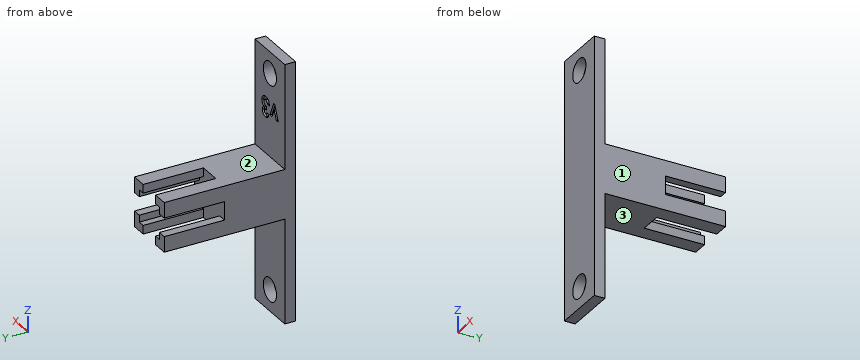
```python
from build123d import *

# Parameters (mm, degrees)
BOSS_EXTRUDE1_DEPTH   = 17.78
BOSS_EXTRUDE1_2_DEPTH = 17.78
BOSS_EXTRUDE1_3_DEPTH = 17.78
BOSS_EXTRUDE1_4_DEPTH = 17.78
SKETCH2_W             = 15.58
SKETCH2_H             = 14.58
BOSS_EXTRUDE2_DEPTH   = 17.78
SKETCH3_W             = 15.58
SKETCH3_H             = 76.2
SKETCH3_R             = 3.429
BOSS_EXTRUDE3_DEPTH   = 3.175
CUT_EXTRUDE3_DEPTH    = 0.635


with BuildPart() as part:
    # Sketch1 → Boss-Extrude1 (new body)
    with BuildSketch(Plane(origin=(0, 0, 0), x_dir=(1, 0, 0), z_dir=(0, 1, 0))):
        Polygon((-5.25, 4.75), (-5.25, 2.718), (-7.79, 2.718), (-7.79, 7.29), (-3.218, 7.29), (-3.218, 4.75), align=None)
    extrude(amount=BOSS_EXTRUDE1_DEPTH)



with BuildPart() as body_2:
    # Sketch1 → Boss-Extrude1 2 (new body)
    with BuildSketch(Plane(origin=(0, 0, 0), x_dir=(1, 0, 0), z_dir=(0, 1, 0))):
        Polygon((7.79, 2.718), (7.79, 7.29), (3.218, 7.29), (3.218, 4.75), (5.25, 4.75), (5.25, 2.718), align=None)
    extrude(amount=BOSS_EXTRUDE1_2_DEPTH)


with BuildPart() as body_3:
    # Sketch1 → Boss-Extrude1 3 (new body)
    with BuildSketch(Plane(origin=(0, 0, 0), x_dir=(1, 0, 0), z_dir=(0, 1, 0))):
        Polygon((5.25, -2.718), (7.79, -2.718), (7.79, -7.29), (3.218, -7.29), (3.218, -4.75), (5.25, -4.75), align=None)
    extrude(amount=BOSS_EXTRUDE1_3_DEPTH)


with BuildPart() as body_4:
    # Sketch1 → Boss-Extrude1 4 (new body)
    with BuildSketch(Plane(origin=(0, 0, 0), x_dir=(1, 0, 0), z_dir=(0, 1, 0))):
        Polygon((-5.25, -2.718), (-7.79, -2.718), (-7.79, -7.29), (-3.218, -7.29), (-3.218, -4.75), (-5.25, -4.75), align=None)
    extrude(amount=BOSS_EXTRUDE1_4_DEPTH)


with BuildPart() as part_1:
    add(part.part)

    add(body_2.part)  # Boss-Extrude2 merges body 2

    add(body_3.part)  # Boss-Extrude2 merges body 3

    add(body_4.part)  # Boss-Extrude2 merges body 4
    # Sketch2 → Boss-Extrude2 (add)
    with BuildSketch(Plane(origin=(0, 0, 0), x_dir=(-1, 0, 0), z_dir=(0, -1, 0))):
        Rectangle(SKETCH2_W, SKETCH2_H)
    extrude(amount=BOSS_EXTRUDE2_DEPTH)

    # Sketch3 → Boss-Extrude3 (add)
    with BuildSketch(Plane(origin=(0, -17.78, 0), x_dir=(-1, 0, 0), z_dir=(0, -1, 0))):
        Rectangle(SKETCH3_W, SKETCH3_H)
        with Locations(Location((0, 31.75, 0), (0, 0, 90))):
            Circle(SKETCH3_R, mode=Mode.SUBTRACT)
        with Locations(Location((0, -31.75, 0), (0, 0, 270))):
            Circle(SKETCH3_R, mode=Mode.SUBTRACT)
    extrude(amount=BOSS_EXTRUDE3_DEPTH)

    # Sketch5 → Cut-Extrude3 (cut)
    with BuildSketch(Plane(origin=(0, -17.78, 0), x_dir=(1, 0, 0), z_dir=(0, 1, 0))):
        Polygon((-4.402938034, -19.56265828), (-3.33951656, -19.56265828), (-2.238782051, -22.073125862), (-1.138047543, -19.56265828), (-0.074626068, -19.56265828), (-1.937945713, -23.816344178), (-2.539618389, -23.816344178), align=None)
        with BuildLine():
            Line((1.60446047, -19.413406143), (0.559695513, -19.413406143))
            add(Edge.make_bspline(
                [(0.559695513, -19.413406143), (0.567071951, -19.36118207), (0.581532969, -19.258800234), (0.616136251, -19.110576841), (0.65752551, -18.969976808), (0.709197886, -18.837445387), (0.769801176, -18.712746497), (0.838719113, -18.59545223), (0.916696725, -18.486066037), (0.976467391, -18.42017136), (1.006285891, -18.387297703)],
                knots=[0, 0, 0, 0, 1.111473889, 2.178970933, 3.205615836, 4.199322666, 5.174200091, 6.12565194, 7.064921805, 8, 8, 8, 8], degree=3))
            add(Edge.make_bspline(
                [(1.006285891, -18.387297703), (1.049295125, -18.343923295), (1.134061806, -18.258436894), (1.275716871, -18.148938257), (1.424197539, -18.054174633), (1.582481657, -17.979045347), (1.748106202, -17.918236894), (1.922388279, -17.877391718), (2.104615709, -17.850290583), (2.228963005, -17.847621027), (2.292419538, -17.846258707)],
                knots=[0, 0, 0, 0, 1.01925491, 2.00884431, 2.983262333, 3.955970413, 4.92937149, 5.924503185, 6.940838805, 8, 8, 8, 8], degree=3))
            add(Edge.make_bspline(
                [(2.292419538, -17.846258707), (2.34883566, -17.847590582), (2.459738389, -17.850208778), (2.622737494, -17.871226235), (2.778143501, -17.908088515), (2.927599095, -17.956285119), (3.068906271, -18.021864654), (3.205183817, -18.097988535), (3.332624133, -18.19135764), (3.451525404, -18.296855331), (3.5607589, -18.410961412), (3.655355585, -18.532931428), (3.736682053, -18.65950728), (3.803684306, -18.791740573), (3.855199933, -18.929855061), (3.890953306, -19.073052878), (3.914354757, -19.221018044), (3.916686153, -19.321587975), (3.91786859, -19.372595012)],
                knots=[0, 0, 0, 0, 1.091422571, 2.145516843, 3.172569842, 4.178562979, 5.178154469, 6.181868002, 7.194278174, 8.227918432, 9.254613415, 10.245994977, 11.209837596, 12.161663635, 13.10878368, 14.055455738, 15.013766427, 16, 16, 16, 16], degree=3))
            add(Edge.make_bspline(
                [(3.91786859, -19.372595012), (3.915442158, -19.435762981), (3.910665261, -19.56012129), (3.871467362, -19.742128915), (3.810111989, -19.916160685), (3.721478187, -20.079781634), (3.610663359, -20.232546477), (3.474697276, -20.369347828), (3.317452606, -20.492330546), (3.199406937, -20.558421473), (3.138959001, -20.592264817)],
                knots=[0, 0, 0, 0, 0.992805628, 1.954529043, 2.915727527, 3.886831945, 4.871318353, 5.87440735, 6.911542536, 8, 8, 8, 8], degree=3))
            add(Edge.make_bspline(
                [(3.138959001, -20.592264817), (3.180449537, -20.605887034), (3.26197658, -20.632654079), (3.377857468, -20.68537147), (3.488046952, -20.742982841), (3.590647607, -20.809912067), (3.686679921, -20.883452827), (3.775558471, -20.964233774), (3.857814283, -21.052078768), (3.932104567, -21.147470922), (3.998040097, -21.248884626), (4.057200536, -21.353977283), (4.105892876, -21.464342641), (4.14714135, -21.578720254), (4.178545589, -21.698138088), (4.20065698, -21.822133409), (4.213437907, -21.950423374), (4.215387216, -22.037339748), (4.216372863, -22.081288088)],
                knots=[0, 0, 0, 0, 1.059543567, 2.081955587, 3.086750234, 4.076226789, 5.052108497, 6.020845489, 6.989030705, 7.970690546, 8.952259656, 9.923888338, 10.895517021, 11.877585046, 12.873342345, 13.889638361, 14.932918083, 16, 16, 16, 16], degree=3))
            add(Edge.make_bspline(
                [(4.216372863, -22.081288088), (4.214374823, -22.145874304), (4.210435096, -22.273225169), (4.18538815, -22.460799959), (4.13875525, -22.639635857), (4.077407087, -22.811790639), (3.995575297, -22.975041849), (3.899273036, -23.13313588), (3.780898209, -23.280590074), (3.649344914, -23.421302739), (3.503247311, -23.549232393), (3.344853741, -23.660141646), (3.177647143, -23.755321519), (3.00056965, -23.832591251), (2.81368278, -23.892097783), (2.61740309, -23.935111847), (2.410905865, -23.961428562), (2.269955352, -23.964187371), (2.19797092, -23.965596314)],
                knots=[0, 0, 0, 0, 1.005138573, 1.981928558, 2.936866704, 3.876260664, 4.820238198, 5.773547, 6.751179199, 7.756627054, 8.768222608, 9.766606018, 10.760583154, 11.757261445, 12.767156078, 13.807575856, 14.880313354, 16, 16, 16, 16], degree=3))
            add(Edge.make_bspline(
                [(2.19797092, -23.965596314), (2.129874809, -23.964110822), (1.996721873, -23.961206138), (1.801957838, -23.936064626), (1.616853058, -23.895509328), (1.440935143, -23.838343272), (1.274884705, -23.764208666), (1.117195935, -23.675930985), (0.971015477, -23.568418577), (0.834714593, -23.446524755), (0.711316847, -23.309766808), (0.601028322, -23.161312666), (0.506280899, -23.000597819), (0.426686017, -22.828308906), (0.362865929, -22.644143683), (0.31252483, -22.448476657), (0.277360749, -22.240925557), (0.266651455, -22.098125985), (0.261191239, -22.025318537)],
                knots=[0, 0, 0, 0, 1.066544725, 2.085487077, 3.070979577, 4.031932826, 4.977951092, 5.916076795, 6.857635327, 7.814973522, 8.776389752, 9.738577119, 10.707772778, 11.69409279, 12.707140348, 13.757286496, 14.856535458, 16, 16, 16, 16], degree=3))
            Line((0.261191239, -22.025318537), (1.305956197, -22.025318537))
            add(Edge.make_bspline(
                [(1.305956197, -22.025318537), (1.312576763, -22.061927077), (1.325472053, -22.133231811), (1.350623524, -22.236465214), (1.383399401, -22.331756021), (1.421296469, -22.419951174), (1.462231007, -22.502208645), (1.511689719, -22.575490462), (1.566048529, -22.641786528), (1.644488688, -22.72060002), (1.756624298, -22.801577594), (1.908044521, -22.871950958), (2.076485181, -22.913198395), (2.194242, -22.918230456), (2.255106504, -22.920831357)],
                knots=[0, 0, 0, 0, 0.928156231, 1.807827665, 2.648129825, 3.438902246, 4.202261636, 4.936546065, 5.639352463, 6.338805438, 7.70633318, 9.064371875, 10.482673459, 12, 12, 12, 12], degree=3))
            add(Edge.make_bspline(
                [(2.255106504, -22.920831357), (2.287403361, -22.92027752), (2.350665678, -22.919192676), (2.443588602, -22.907168637), (2.53211077, -22.887365035), (2.616397061, -22.860452674), (2.696984046, -22.826716347), (2.772332028, -22.783215372), (2.84397679, -22.732639278), (2.911139487, -22.675778323), (2.973199203, -22.613820236), (3.024836536, -22.545212181), (3.072029323, -22.475494135), (3.106933447, -22.400104897), (3.13751698, -22.323101214), (3.156235665, -22.241688093), (3.170369616, -22.157573363), (3.171191024, -22.100008934), (3.171607906, -22.070793797)],
                knots=[0, 0, 0, 0, 1.110435564, 2.175094844, 3.216326037, 4.226890168, 5.215276772, 6.21526065, 7.213097102, 8.228249917, 9.239874822, 10.221364777, 11.178138315, 12.128914389, 13.072518965, 14.022636769, 14.996447288, 16, 16, 16, 16], degree=3))
            add(Edge.make_bspline(
                [(3.171607906, -22.070793797), (3.170501163, -22.038842067), (3.168297891, -21.975233493), (3.150296928, -21.882410155), (3.121869603, -21.793121585), (3.082380576, -21.707763195), (3.029647382, -21.626649598), (2.9674228, -21.548153411), (2.890804565, -21.47636022), (2.806744099, -21.405394826), (2.709266982, -21.343534406), (2.603120486, -21.286446328), (2.485514916, -21.241021842), (2.35932113, -21.200449362), (2.222152054, -21.170815853), (2.074859456, -21.149299038), (1.917680943, -21.133283103), (1.809335751, -21.130985354), (1.753712607, -21.129805716)],
                knots=[0, 0, 0, 0, 0.809814727, 1.612155564, 2.388397, 3.182215007, 3.988903953, 4.837162975, 5.715530372, 6.646997145, 7.623086902, 8.637258368, 9.698941581, 10.815059213, 11.996518529, 13.252603015, 14.589518788, 16, 16, 16, 16], degree=3))
            Line((1.753712607, -21.129805716), (1.753712607, -20.159666827))
            add(Edge.make_bspline(
                [(1.753712607, -20.159666827), (1.822966729, -20.153768925), (1.952527477, -20.142735117), (2.132364742, -20.116932174), (2.283764537, -20.082442292), (2.410365759, -20.040832116), (2.515487302, -19.98739381), (2.607320901, -19.92840028), (2.686412341, -19.859887916), (2.753255217, -19.783899748), (2.806727438, -19.702295581), (2.844571961, -19.616343786), (2.869562507, -19.528703818), (2.871930359, -19.468760721), (2.873103632, -19.439058854)],
                knots=[0, 0, 0, 0, 1.70044513, 3.18119609, 4.440695891, 5.496282586, 6.431922213, 7.318171381, 8.16090191, 8.983045123, 9.787564368, 10.536848927, 11.275007137, 12, 12, 12, 12], degree=3))
            add(Edge.make_bspline(
                [(2.873103632, -19.439058854), (2.8710794, -19.401162498), (2.867128528, -19.327196833), (2.83644391, -19.221336386), (2.783178889, -19.126970571), (2.71175985, -19.044297961), (2.624733268, -18.975243601), (2.522722857, -18.925111313), (2.40794225, -18.895656355), (2.327187908, -18.892602868), (2.285423344, -18.891023665)],
                knots=[0, 0, 0, 0, 1.009664648, 1.970651636, 2.907870547, 3.878035693, 4.867062054, 5.849714035, 6.887914197, 8, 8, 8, 8], degree=3))
            add(Edge.make_bspline(
                [(2.285423344, -18.891023665), (2.247568462, -18.892886959), (2.172452782, -18.896584305), (2.062611175, -18.924180317), (1.958298243, -18.970634769), (1.861674014, -19.03469272), (1.774133277, -19.111623605), (1.702287588, -19.202732269), (1.642529751, -19.302560235), (1.617199978, -19.376312658), (1.60446047, -19.413406143)],
                knots=[0, 0, 0, 0, 0.98818071, 1.960853194, 2.938124878, 3.957524365, 4.978590984, 5.968022688, 6.978025184, 8, 8, 8, 8], degree=3))
        make_face()
    extrude(amount=-CUT_EXTRUDE3_DEPTH, mode=Mode.SUBTRACT)


solid = part_1.part
```
Input: part model. Units: mm. Frame: model coordinates. Face numbers are marked on the shaded views. A direction names the side the tool comes from. Round coordinates to 2 decimals unless told otherwise and drop trailing zeros. Loops run counter-clockwise (first coordinate to the right, second up) from the corner with the lowest first, then second, coordinate; pieces in that order, holes last. Notation, with made-up numbers: (12.5, -10.5) - (21.5, -10.5) arc R26 ccw to (21.5, 24.5) - close; hole circle Ø8 at (55.25, 28). An arc over 180 degrees is marked (long way). One line per item, written item: value. Start each with the question number.
(1) Ray query, line 1 (X direction, y = -18.8, z = -31.75); line 2 (Z direction, x = 7, y = 15); line 3 (Z direction, x = -5, y = 5.5). Return the intervals inside material, ascending. Write a range as [from, to].
(2) Section A-A, the plane z = -31.75. Return loops of the section in (x, y) (3 decimals).
(3) Section C-C, the plane x = -6.25. Return loops of the section in (y, z) (3 decimals), plus the area to 3 significant figures.
(4) Section D-D, the plane z = 2. Return loops of the section in (x, y) (3 decimals), plus the area to 3 significant figures.
(5) Contact query for flat-ended pins moving along their axis: P1, Ø0.8, axis at x = -7, y = 5.5, coming from the -Z side; P2, Ø1.2, axis at x = 2.5, z = 20, coming from the +Y side; P3, Ø3, axis at x = -7, y = 9, coming from the +Z side. Output: stop coordinate, or through.
(6) Access query for the marked faces 1, 2 and 3. Directions: +Z, -Z, +X, -X, +Y, -Y. A direction counts if a zero-diameter tool reaches every point of the face in a straight line with its end or side. Return the directions, or none.
(7) Section B-B, the plane y = 14. Return loops of the section in (x, z), plus the area to 3 significant figures.
Results below:
1. line 1: [-7.79, -3.43], [3.43, 7.79]
1. line 2: [-7.29, -2.72], [2.72, 7.29]
1. line 3: [-7.29, -4.75], [4.75, 7.29]
2. outline: (-7.79, -20.955) - (-3.429, -20.955) - (-3.429, -17.78) - (-7.79, -17.78) - close; (3.429, -20.955) - (7.79, -20.955) - (7.79, -17.78) - (3.429, -17.78) - close
3. outline: (-20.955, -38.1) - (-17.78, -38.1) - (-17.78, -7.29) - (17.78, -7.29) - (17.78, -2.718) - (0, -2.718) - (0, 2.718) - (17.78, 2.718) - (17.78, 7.29) - (-17.78, 7.29) - (-17.78, 38.1) - (-20.955, 38.1) - close
3. area: 664 mm^2
4. outline: (-7.79, -20.955) - (7.79, -20.955) - (7.79, 0) - (-7.79, 0) - close
4. area: 326 mm^2
5. P1: z = -7.29
5. P2: y = -17.78
5. P3: z = 7.29
6. face 1: +Z, -Z, +X, +Y, -Y
6. face 2: +Z, +X, -X, +Y
6. face 3: -Z, +X, -X, +Y
7. outline: (-7.79, -7.29) - (-3.22, -7.29) - (-3.22, -4.75) - (-5.25, -4.75) - (-5.25, -2.72) - (-7.79, -2.72) - close; (-7.79, 2.72) - (-5.25, 2.72) - (-5.25, 4.75) - (-3.22, 4.75) - (-3.22, 7.29) - (-7.79, 7.29) - close; (3.22, -7.29) - (7.79, -7.29) - (7.79, -2.72) - (5.25, -2.72) - (5.25, -4.75) - (3.22, -4.75) - close; (3.22, 4.75) - (5.25, 4.75) - (5.25, 2.72) - (7.79, 2.72) - (7.79, 7.29) - (3.22, 7.29) - close
7. area: 67.1 mm^2
